Model file for the job. Use its own axes, mm. Face numbers are marked on the shaded views. A direction names the side the tool comes from. Coordinates: 2 decimals unless noted, no trailing zeros. Order: outer loops, then holes, each group sorted by start corner. A loop starts at its lowest first (then second) coordinate and runs counter-clockwise, first axis right, second up.
from build123d import *

# Parameters (mm, degrees)
F0_R     = 1.5
F1_DEPTH = 15
F2_W     = 60.5
F2_H     = 8
F3_DEPTH = 5
F4_W     = 22
F4_H     = 3
F5_DEPTH = 120
F6_R     = 1
F7_R     = 1
F8_R     = 1


with BuildPart() as f1:
    # F0 (on Top) → F1 (new body)
    with BuildSketch(Plane.XY):
        with BuildLine():
            Line((18, 12.5), (0, 12.5))
            Line((0, 12.5), (0, -12.5))
            Line((0, -12.5), (18, -12.5))
            Line((18, -12.5), (18, -11))
            Line((18, -11), (14, -11))
            ThreePointArc((14, -11), (13.292893, -10.707107), (13, -10))
            Line((13, -10), (13, 10))
            ThreePointArc((13, 10), (13.292893, 10.707107), (14, 11))
            Line((14, 11), (18, 11))
            Line((18, 11), (18, 12.5))
        make_face()
        with BuildLine():
            ThreePointArc((1.5, 10), (1.792893, 10.707107), (2.5, 11))
            Line((2.5, 11), (5.5, 11))
            ThreePointArc((5.5, 11), (6.207107, 10.707107), (6.5, 10))
            Line((6.5, 10), (6.5, -10))
            ThreePointArc((6.5, -10), (6.207107, -10.707107), (5.5, -11))
            Line((5.5, -11), (2.5, -11))
            ThreePointArc((2.5, -11), (1.792893, -10.707107), (1.5, -10))
            Line((1.5, -10), (1.5, 10))
        make_face(mode=Mode.SUBTRACT)
        with Locations((9.75, 0)):
            Circle(F0_R, mode=Mode.SUBTRACT)
        with BuildLine():
            Line((36, 12.5), (18, 12.5))
            Line((18, 12.5), (18, 11))
            Line((18, 11), (18, -11))
            Line((18, -11), (18, -12.5))
            Line((18, -12.5), (36, -12.5))
            Line((36, -12.5), (36, -11))
            Line((36, -11), (32, -11))
            ThreePointArc((32, -11), (31.292893, -10.707107), (31, -10))
            Line((31, -10), (31, 10))
            ThreePointArc((31, 10), (31.292893, 10.707107), (32, 11))
            Line((32, 11), (36, 11))
            Line((36, 11), (36, 12.5))
        make_face()
        with BuildLine():
            ThreePointArc((23.5, 11), (24.207107, 10.707107), (24.5, 10))
            Line((24.5, 10), (24.5, -10))
            ThreePointArc((24.5, -10), (24.207107, -10.707107), (23.5, -11))
            Line((23.5, -11), (20.5, -11))
            ThreePointArc((20.5, -11), (19.792893, -10.707107), (19.5, -10))
            Line((19.5, -10), (19.5, 10))
            ThreePointArc((19.5, 10), (19.792893, 10.707107), (20.5, 11))
            Line((20.5, 11), (23.5, 11))
        make_face(mode=Mode.SUBTRACT)
        with Locations((27.75, 0)):
            Circle(F0_R, mode=Mode.SUBTRACT)
        with BuildLine():
            Line((54, 12.5), (36, 12.5))
            Line((36, 12.5), (36, 11))
            Line((36, 11), (36, -11))
            Line((36, -11), (36, -12.5))
            Line((36, -12.5), (54, -12.5))
            Line((54, -12.5), (54, -11))
            Line((54, -11), (50, -11))
            ThreePointArc((50, -11), (49.292893, -10.707107), (49, -10))
            Line((49, -10), (49, 10))
            ThreePointArc((49, 10), (49.292893, 10.707107), (50, 11))
            Line((50, 11), (54, 11))
            Line((54, 11), (54, 12.5))
        make_face()
        with BuildLine():
            ThreePointArc((41.5, 11), (42.207107, 10.707107), (42.5, 10))
            Line((42.5, 10), (42.5, -10))
            ThreePointArc((42.5, -10), (42.207107, -10.707107), (41.5, -11))
            Line((41.5, -11), (38.5, -11))
            ThreePointArc((38.5, -11), (37.792893, -10.707107), (37.5, -10))
            Line((37.5, -10), (37.5, 10))
            ThreePointArc((37.5, 10), (37.792893, 10.707107), (38.5, 11))
            Line((38.5, 11), (41.5, 11))
        make_face(mode=Mode.SUBTRACT)
        with Locations((45.75, 0)):
            Circle(F0_R, mode=Mode.SUBTRACT)
        with BuildLine():
            Line((72, 12.5), (54, 12.5))
            Line((54, 12.5), (54, 11))
            Line((54, 11), (54, -11))
            Line((54, -11), (54, -12.5))
            Line((54, -12.5), (72, -12.5))
            Line((72, -12.5), (72, -11))
            Line((72, -11), (68, -11))
            ThreePointArc((68, -11), (67.292893, -10.707107), (67, -10))
            Line((67, -10), (67, 10))
            ThreePointArc((67, 10), (67.292893, 10.707107), (68, 11))
            Line((68, 11), (72, 11))
            Line((72, 11), (72, 12.5))
        make_face()
        with BuildLine():
            ThreePointArc((59.5, 11), (60.207107, 10.707107), (60.5, 10))
            Line((60.5, 10), (60.5, -10))
            ThreePointArc((60.5, -10), (60.207107, -10.707107), (59.5, -11))
            Line((59.5, -11), (56.5, -11))
            ThreePointArc((56.5, -11), (55.792893, -10.707107), (55.5, -10))
            Line((55.5, -10), (55.5, 10))
            ThreePointArc((55.5, 10), (55.792893, 10.707107), (56.5, 11))
            Line((56.5, 11), (59.5, 11))
        make_face(mode=Mode.SUBTRACT)
    extrude(amount=F1_DEPTH)

    # F2 (on Top) → F3 (cut)
    with BuildSketch(Plane.XY):
        with Locations((36.75, 0)):
            Rectangle(F2_W, F2_H)
    extrude(amount=F3_DEPTH, mode=Mode.SUBTRACT)

    # F4 (on face) → F5 (cut)
    with BuildSketch(Plane(origin=(0, 0, 0), x_dir=(0, -1, 0), z_dir=(-1, 0, 0))):
        with Locations((0, 13.5)):
            Rectangle(F4_W, F4_H)
    extrude(amount=-F5_DEPTH, mode=Mode.SUBTRACT)

    # F6
    f6_edges = [f1.edges().sort_by_distance(p)[0] for p in [
        (54, 11, 6),
        (36, 11, 6),
        (54, -11, 6),
        (36, -11, 6),
    ]]
    fillet(f6_edges, radius=F6_R)

    # F7
    f7_edges = [f1.edges().sort_by_distance(p)[0] for p in [
        (18, 11, 6),
    ]]
    fillet(f7_edges, radius=F7_R)

    # F8
    f8_edges = [f1.edges().sort_by_distance(p)[0] for p in [
        (18, -11, 6),
    ]]
    fillet(f8_edges, radius=F8_R)


solid = f1.part
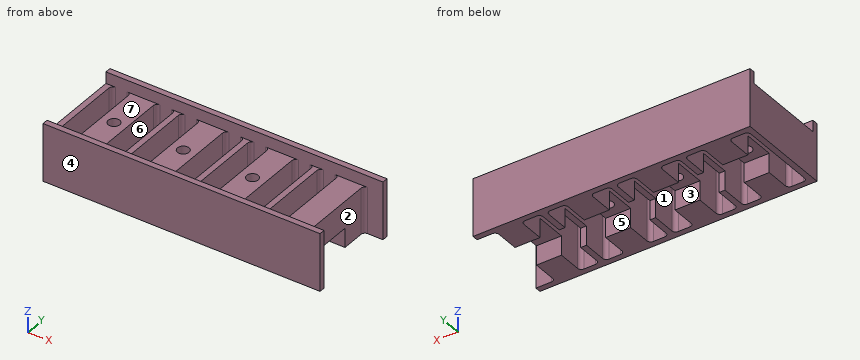
Q1. Probe line 1 (Y direction, x = 68, z = 12); line 2 (Y direction, x = 27.75, z = 10); line 3 (Z direction, x = 66.5, y = 10). List the from-to ranges inside material, lowest first.
Established:
line 1: y = -12.5 to -11, 11 to 12.5
line 2: y = -12.5 to -1.5, 1.5 to 12.5
line 3: z = 0 to 12
Q2. Cut at B-B, the plane x = 27.75. List the corners of the cut face in (y, z), plus the area to 3 significant figures.
Established:
outline: (-12.5, 0) - (-4, 0) - (-4, 5) - (-1.5, 5) - (-1.5, 12) - (-11, 12) - (-11, 15) - (-12.5, 15) - close; (1.5, 5) - (4, 5) - (4, 0) - (12.5, 0) - (12.5, 15) - (11, 15) - (11, 12) - (1.5, 12) - close
area: 248 mm2
Q3. Drop flat-ended pins along their axis: P1, Ø6, axis at y = -3, z = 6.5, coming from the +X side; P2, Ø4, axis at x = 55.5, y = -0.5, coming from the +Z side; P3, Ø2, axis at y = 2, z = 2.5, coming from the +X side. Give the stop position or say it passes through.
Established:
P1: stops at x = 67
P2: stops at z = 12
P3: stops at x = 1.5
Q4. Cut at A-A, the plane y = 6.5. Count the separate pieces of the cut face and the enclosed holes in it, plus the area to 3 significant figures.
Established:
separate pieces: 8
enclosed holes: 0
area: 384 mm2
Q5. Mould opens along X. For the marked faces 1, 2 and 3 say: pulls with the +X half, pulls with the -X half, needs draft (parallel to the pull), parting line crosses it, or undercut.
Established:
face 1: undercut
face 2: pulls with the +X half
face 3: needs draft
Q6. Which spindle directions (+Z, -Z, +X, -X, +Y, -Y) get a long thin tool onto all of the face, cutting with end or side? Do the marked faces 4, 5, 6 and 7. Say none if no direction does.
Established:
face 4: +Z, -Z, +X, -X, -Y
face 5: -Z, +X
face 6: +Z, -Z
face 7: +Z, +X, -X
